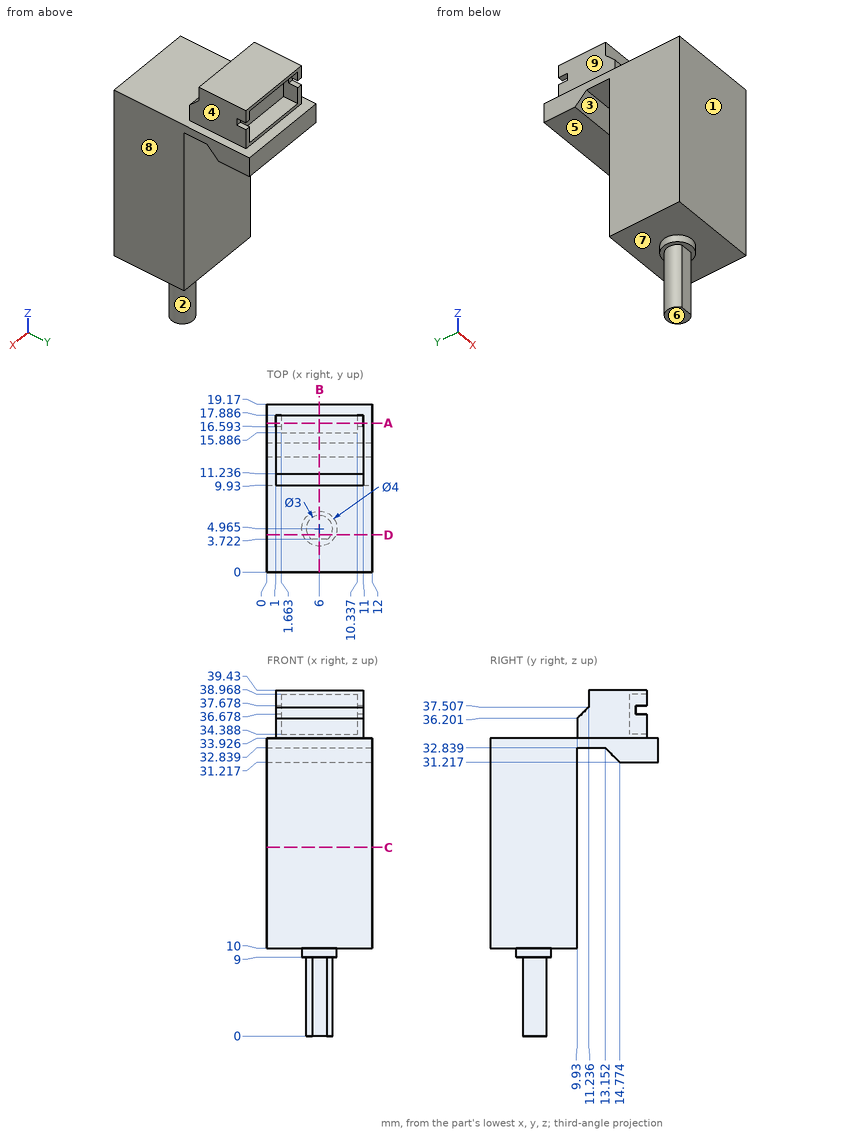
Could you check a few things on this drawing? It's one solid part, dimensions in mm from its lowest x, y, z. A direction names the side the tool comes from. Give positions to 0.01 mm unless a question says otherwise; leave off trailing zeros. Loops run counter-clockwise (first coordinate to the right, second up) from the corner with the lowest first, then second, coordinate; pieces in that order, holes last. Notation, with made-up numbers: M 36.25,24.5 L 42.25,24.5 A22 cw 42.25,32.5 Z; hole C 85,-39.75 d11. An arc over 180 degrees is marked long. Return JSON: item names as keys, results as strings.
Item 1: Imagine slicing it at C-C on z = 21.5. List the corners of the cut face in (x, y) for me.
A:
{"outline": "M 0,0 L 12,0 L 12,9.93 L 0,9.93 Z"}
Item 2: Imagine slicing it at D-D on y = 4.25. List the corners of the cut face in (x, z) for me, then the cut area to 3 significant figures.
A:
{"outline": "M 0,10 L 4.13,10 L 4.13,9 L 4.68,9 L 4.68,0 L 7.32,0 L 7.32,9 L 7.87,9 L 7.87,10 L 12,10 L 12,33.93 L 0,33.93 Z", "area": "315 mm^2"}
Item 3: Thinking about a two-plate mould opening in Y: for the marked faces 1, 2, 3 and 4, which applies, released by +Y, released by -Y, zero draft, split by the parting line, or undercut?
A:
{"face 1": "released by -Y", "face 2": "split by the parting line", "face 3": "undercut", "face 4": "zero draft"}
Item 4: On a 3-axis mill with a long thin cutter (end or side, diameter ignored), from which of +Z, -Z, +X, -X, +Y, -Y can I reach the whole of each face in a straight line? I mean the marked faces 5, 6, 7, 8 and 9. Say none if no direction works.
A:
{"face 5": "-Z, +X, -X, +Y", "face 6": "-Z, +X, -X, +Y, -Y", "face 7": "-Z", "face 8": "+Z, -Z, +X, +Y, -Y", "face 9": "+Z, -X, +Y, -Y"}
Item 5: Imagine slicing it at A-A on y = 17. List the corners of the cut face in (x, z) for me.
A:
{"outline": "M 0,31.22 L 12,31.22 L 12,33.93 L 11,33.93 L 11,36.68 L 10.34,36.68 L 10.34,34.39 L 1.66,34.39 L 1.66,36.68 L 1,36.68 L 1,33.93 L 0,33.93 Z; M 1,37.68 L 1.66,37.68 L 1.66,38.97 L 10.34,38.97 L 10.34,37.68 L 11,37.68 L 11,39.43 L 1,39.43 Z"}
Item 6: Imagine slicing it at B-B on x = 6. List the corners of the cut face in (y, z) for me (1 decimal), then the cut area to 3 significant figures.
A:
{"outline": "M 0,10 L 3,10 L 3,9 L 3.7,9 L 3.7,0 L 6.5,0 L 6.5,9 L 7,9 L 7,10 L 9.9,10 L 9.9,32.8 L 13.2,32.8 L 14.8,31.2 L 19.2,31.2 L 19.2,33.9 L 17.9,33.9 L 17.9,34.4 L 15.9,34.4 L 15.9,39 L 17.9,39 L 17.9,39.4 L 11.2,39.4 L 11.2,37.5 L 9.9,36.2 L 9.9,33.9 L 0,33.9 Z", "area": "316 mm^2"}
Item 7: Please list where these lines run through material, in increasing order: line 1 (Z direction, x = 4, y = 17); line 2 (Z direction, x = 10.5, y = 16.75); line 3 (Z direction, x = 2.25, y = 18).
A:
{"line 1": "z = 31.22 to 34.39, 38.97 to 39.43", "line 2": "z = 31.22 to 36.68, 37.68 to 39.43", "line 3": "z = 31.22 to 33.93"}
Item 8: I'm going to push flat-ended pins straight in: pin 1 Ø0.5 at (x, z) = (5.5, 3.5) entering from -Y; pin 2 Ø6 at (x, y) = (9, 10.5) entering from +Z; pin 3 Ø1 at (y, z) = (4.5, 35.5) entering from +X; pin 4 Ø1.1 at (x, z) = (5.5, 35) entering from -Y. Where does each tip first touch, or does it pass through?
A:
{"pin 1": "stops at y = 3.72", "pin 2": "stops at z = 39.43", "pin 3": "passes through", "pin 4": "stops at y = 9.93"}
